Could you check a few things on this model? Use its own coordinates, in mm. Face numbers are marked on the shaded views. A direction names the side the tool comes from. Round coordinates to 2 decimals unless told otherwise and drop trailing zeros. Order: outer loops, then holes, each group sorted by start corner. A loop starts at its lowest first (then second) coordinate and runs counter-clockwise, first axis right, second up. Notation, with made-up numbers: M 25,-4 L 40,-4 A17 cw 40,14 Z; hole C 58,-9.75 d7. An arc over 180 degrees is marked long. Write each question's results on one line, items separated by ' | '. Start each with the question number.
1. Suppose I cut it at B-B on z = -26.75. Write out the boundary of the cut face in (x, y), and give its area (3 significant figures).
2. We'd pull the mould along Y, two halves only. Please class the marked faces 4, 5 and 6: released by +Y, released by -Y, zero draft, split by the parting line, or undercut.
3. Suppose I cut it at C-C on x = 17.5. Write out the boundary of the cut face in (y, z), and give its area (3 significant figures).
4. Suppose I cut it at A-A on y = 6.56. Write out the boundary of the cut face in (x, z).
5. Please list where these lines run through material, in increasing order: L1, parallel to Y at x = 21.45, z = -15 (1 decimal); L2, parallel to Y at x = 28, z = -15 (3 decimals); L3, parallel to Z at x = 11.5, y = 28.
6. Suppose I cut it at D-D on z = -15. Give the number of separate pieces and of enclosed holes in the cut face, and give its area (3 significant figures).
7. For the marked faces 1, 2 and 3, which set-ups out of +Z, -Z, +X, -X, +Y, -Y let a thin tool reach every point of the face, with its end or its side?
8. I'm going to push flat-ended pins straight in: pin 1 (6 mm diameter, centred on x = 7, z = -17, fed in from -Y); pin 2 (4 mm diameter, centred on x = 10.5, z = -25.5, fed in from -Y); pin 3 (11 mm diameter, centred on x = 25.5, y = -9, fed in from -Z) (3 decimals). Where does each tip first touch, or does it pass through?
Autodesk Inventor part; units mm, degrees
ref_plane "YZ Plane" through (0, 0, 0) normal (1, 0, 0) x (0, 1, 0)
ref_plane "XZ Plane" through (0, 0, 0) normal (0, 1, 0) x (-1, 0, 0)
ref_plane "XY Plane" through (0, 0, 0) normal (0, 0, 1) x (1, 0, 0)
sketch "Sketch1" plane through (0, 0, 0) normal (0, 0, 1) x (1, 0, 0)
  line L0 (0, 0) -> (25, 0)
  line L1 (25, 0) -> (25, 40)
  line L2 (25, 40) -> (0, 40)
  line L3 (0, 40) -> (0, 0)
  dimension "d1" = 25
  dimension "d2" = 40
  dimension "d3" = 25
extrude "Extrusion1" add sketch "Sketch1" against normal blind 30
sketch "Sketch2" plane through (25, 0, 0) normal (1, 0, 0) x (0, 0, -1)
  line L0 (0, 0) -> (30, 0)
  circle A0 centre (15, 6.56) radius 2.46
extrude "Extrusion2" cut sketch "Sketch2" against normal blind 30
sketch "Sketch3" plane through (0, 0, 0) normal (-1, 0, 0) x (0, 0, 1)
  line L0 (0, 0) -> (-30, 0)
  line L1 (-25.05, 0) -> (-4.95, 0)
  line L2 (-4.95, 0) -> (-4.95, 33.12)
  line L3 (-4.95, 33.12) -> (-25.05, 33.12)
  line L4 (-25.05, 33.12) -> (-25.05, 0)
  dimension "d11" = 20.1
extrude "Extrusion3" cut sketch "Sketch3" against normal blind 20
sketch "Sketch4" plane through (0, 0, 0) normal (0, -1, 0) x (1, 0, 0)
  line L0 (20, -4.95) -> (20, -25.05)
  line L1 (20, -15) -> (25, -15)
  line L2 (25, 0) -> (25, -30)
  line L3 (20, -8.025) -> (25, -8.025)
  line L4 (25, -8.025) -> (25, -21.975)
  line L5 (25, -21.975) -> (20, -21.975)
  line L6 (20, -21.975) -> (20, -8.025)
  line L7 (20, -8.025) -> (25, -21.975) construction
  line L8 (25, -8.025) -> (20, -21.975) construction
  line L9 (25, -12.54) -> (25, -17.46)
  point P0 (0, 0)
  point P1 (22.5, -15)
  dimension "d14" = 13.95
extrude "Extrusion4" add sketch "Sketch4" along normal blind 15
sketch "Sketch5" plane through (20, 0, 0) normal (-1, 0, 0) x (0, 0, 1)
  circle A0 centre (-15, 6.56) radius 2.46
  circle A1 centre (-15, 6.56) radius 4.7025
  circle A2 centre (-15, 6.56) radius 2.46
  circle A3 centre (-15, 6.56) radius 2.46
  point P0 (0, 0)
  dimension "d17" = 9.405
extrude "Extrusion5" cut sketch "Sketch5" against normal blind 2.1
sketch "Sketch6" plane through (25, 0, 0) normal (1, 0, 0) x (0, 0, -1)
  circle A0 centre (15, 6.56) radius 4.7025
  line L0 (15, 6.56) -> (15, 23.56)
  circle A1 centre (15, 23.56) radius 2.46
  point P0 (0, 0)
  dimension "d20" = 17
  dimension "d21" = 4.92
extrude "Extrusion6" cut sketch "Sketch6" against normal blind 10 contours A1
sketch "Sketch7" plane through (20, 0, 0) normal (-1, 0, 0) x (0, 0, 1)
  circle A0 centre (-15, 23.56) radius 2.46
  circle A1 centre (-15, 23.56) radius 4.7025
  point P0 (0, 0)
  dimension "d24" = 9.405
extrude "Extrusion7" cut sketch "Sketch7" against normal blind 2.1
sketch "Sketch9" plane through (25, 0, 0) normal (1, 0, 0) x (0, 0, -1)
  circle A0 centre (15, 6.56) radius 2.46
  circle A1 centre (15, 6.56) radius 2.46
  circle A2 centre (15, 23.56) radius 2.46
  circle A3 centre (15, 23.56) radius 2.46
  line L0 (30, 40) -> (30, 0)
  line L1 (30, 0) -> (30, 40)
  line L2 (30, 40) -> (0, 40)
  line L3 (0, 40) -> (0, 0)
  line L4 (0, 0) -> (8.025, 0)
  line L5 (21.975, 0) -> (21.975, -15)
  line L6 (21.975, -15) -> (8.025, -15)
  line L7 (8.025, -15) -> (8.025, 0)
  line L8 (0, 0) -> (8.025, 0)
  line L9 (21.975, 0) -> (30, 0)
extrude "Extrusion8" add sketch "Sketch9" along normal blind 5
sketch "Sketch10" plane through (0, 40, 0) normal (0, 1, 0) x (1, 0, 0)
  line L0 (0, 30) -> (30, 30)
  line L1 (30, 0) -> (0, 0)
  line L2 (0, 30) -> (30, 30)
  line L3 (30, 30) -> (30, 0)
  line L4 (30, 0) -> (0, 0)
  line L5 (0, 0) -> (0, 30)
extrude "Extrusion9" add sketch "Sketch10" along normal blind 30
sketch "Sketch12" plane through (30, 0, 0) normal (1, 0, 0) x (0, 0, -1)
  circle A0 centre (15, 6.56) radius 2.46
  line L0 (15, 6.56) -> (15, 15.06)
  circle A1 centre (15, 15.06) radius 2.525
  point P0 (0, 0)
  dimension "d31" = 8.5
  dimension "d33" = 5.05
extrude "Extrusion10" cut sketch "Sketch12" against normal blind 30 contours A1
sketch "Sketch15" plane through (0, 0, -25.05) normal (-1, 0, 0) x (0, 0, 1)
  line L0 (0, 33.12) -> (20.1, 33.12)
  line L1 (20.1, 33.12) -> (20.1, 0)
  line L2 (0, 33.12) -> (20.1, 33.12)
  line L3 (20.1, 33.12) -> (20.1, 31.1)
  line L4 (20.1, 31.1) -> (0, 31.1)
  line L5 (0, 31.1) -> (0, 33.12)
  point P0 (25.05, 0)
  dimension "d57" = 2.02
extrude "Extrusion13" add sketch "Sketch15" against normal blind 20
sketch "Sketch17" plane through (0, 0, 0) normal (0, 0, 1) x (1, 0, 0)
  line L0 (0, 70) -> (30, 70)
  line L1 (30, 70) -> (50.0622, 90.0622)
  line L2 (30, 70) -> (80, 70) construction
  line L3 (11.9522, 97.2454) -> (0, 85.2932)
  line L4 (0, 70) -> (0, 85.2932)
  line L5 (0, 70) -> (0, 0)
  line L6 (0, 70) -> (30, 70)
  line L7 (10.923, 112.2849) -> (0, 120.567)
  line L8 (50.0622, 105.3553) -> (50.0622, 120.567)
  line L9 (50.0622, 105.3553) -> (50.0622, 90.0622)
  arc A0 (11.9522, 97.2454) -> (10.923, 112.2849) centre (4.8811, 104.3165) ccw
  line L10 (0, 152.567) -> (30, 152.567)
  line L11 (30, 152.567) -> (50.0622, 120.567)
  line L12 (5, 150.567) -> (0, 152.567)
  line L13 (5, 122.567) -> (0, 120.567)
  line L14 (5, 122.567) -> (10, 136.567)
  line L15 (10, 136.567) -> (5, 150.567)
  dimension "d61" = 45
  dimension "d62" = 32.0271
  dimension "d72" = 10
extrude "Extrusion14" add sketch "Sketch17" against normal blind 30
properties part number "rec_c_28mm_x_30mm"
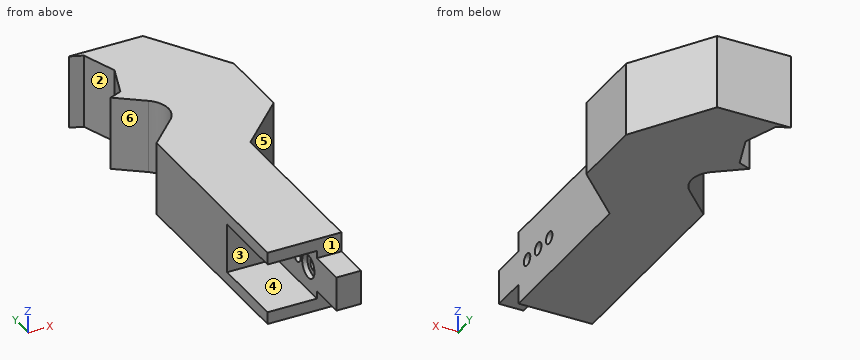
Filled sheet:
1) outline: M 0,0 L 30,0 L 30,70 L 50.06,90.06 L 50.06,120.57 L 30,152.57 L 0,152.57 L 5,150.57 L 10,136.57 L 5,122.57 L 0,120.57 L 10.92,112.28 A10 cw 11.95,97.25 L 0,85.29 Z | area: 5,170 mm^2
2) face 4: zero draft | face 5: released by -Y | face 6: undercut
3) outline: M 0,-30 L 152.57,-30 L 152.57,0 L 0,0 L 0,-4.95 L 31.1,-4.95 L 31.1,-25.05 L 0,-25.05 Z | area: 3,950 mm^2
4) outline: M 0,-30 L 30,-30 L 30,-17.46 L 22.1,-17.46 L 22.1,-19.7 L 20,-19.7 L 20,-25.05 L 0,-25.05 Z; M 0,-4.95 L 20,-4.95 L 20,-10.3 L 22.1,-10.3 L 22.1,-12.54 L 30,-12.54 L 30,0 L 0,0 Z
5) L1: y = -15 to 1.9, 11.3 to 12.5, 17.6 to 18.9, 28.3 to 152.6 | L2: y = -15 to 4.1, 9.02 to 12.535, 17.585 to 21.1, 26.02 to 152.567 | L3: z = -30 to -25.05, -4.95 to 0
6) separate pieces: 4 | enclosed holes: 0 | area: 4,530 mm^2
7) face 1: +Z, +X, -X, -Y | face 2: +Z, -Z, -X | face 3: -X, -Y
8) pin 1: stops at y = 31.1 | pin 2: stops at y = 0 | pin 3: stops at z = -21.975
